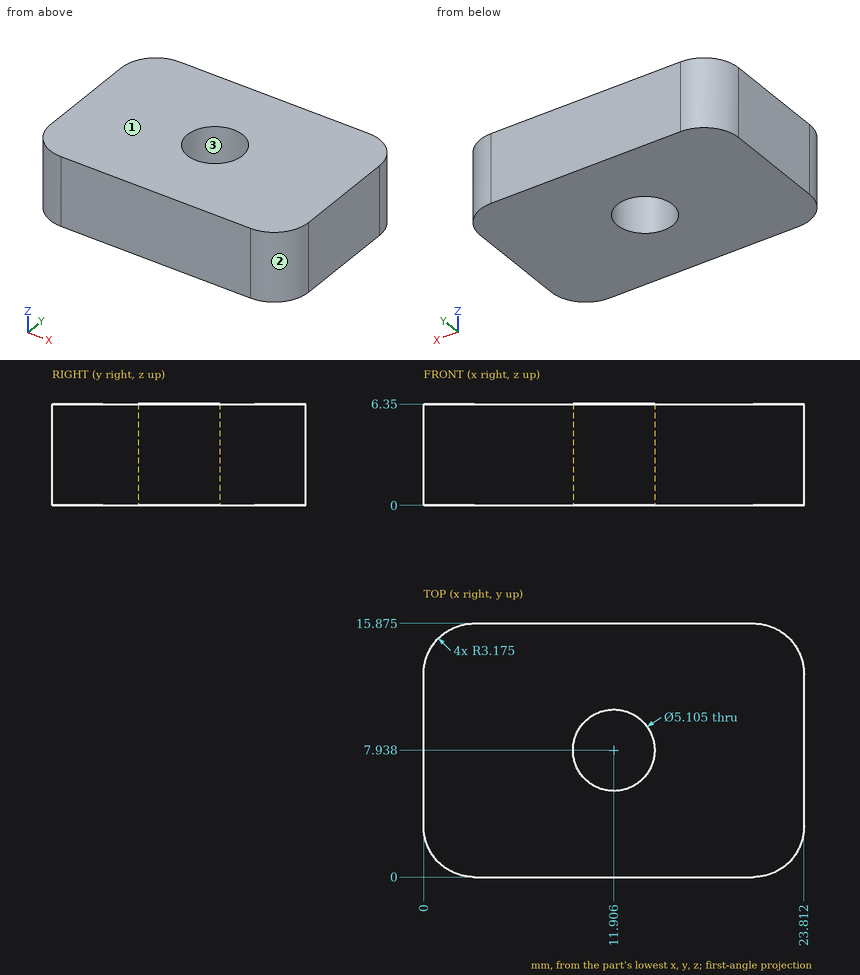
Input: dimensioned drawing with shaded views. Units: mm. Origin: part minimum x, y, z. Give positions to 0.01 mm unless a question says otherwise; leave off trailing zeros. Put each result on its own line as item: value. Start each with the question number.
1) Pull-direction query (X, two-part tool) for the marked faces 1, 2 and 3; classes: pulls with the +X half, pulls with the -X half, needs draft (parallel to the pull), parting line crosses it, or undercut.
2) Ray query, line 1 along Y through (x, z) = (13.5, 0.5) (1 decimal); line 2 along X through (y, z) = (8.75, 2.5) (1 decimal); line 3 along X through (y, z) = (6.5, 1.75) (1 decimal). Return the intervals inside material, ascending.
3) Contact query for a flat-ended pin moving along its axis: pin 1 (6.5 mm diameter, centred on x = 11.91, y = 7.94, fed in from +Z). Output: stop coordinate, or through.
Verdict:
1. face 1: needs draft
1. face 2: pulls with the +X half
1. face 3: undercut
2. line 1: 0 to 5.9, 9.9 to 15.9
2. line 2: 0 to 9.5, 14.3 to 23.8
2. line 3: 0 to 9.8, 14 to 23.8
3. pin 1: z = 6.35
